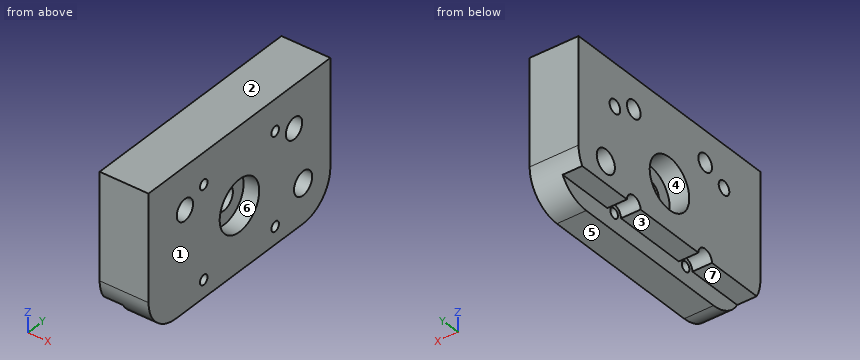
```python
from build123d import *

# Parameters (mm, degrees)
SKETCH_R        = 3.5
SKETCH_R_2      = 6
PAD_DEPTH       = 25
SKETCH001_R     = 5.4
POCKET_DEPTH    = 15
SKETCH002_R     = 13.05
POCKET001_DEPTH = 10
SKETCH006_R     = 2.5
SKETCH006_R_2   = 6
POCKET002_DEPTH = 25
SKETCH005_R     = 4.5
POCKET003_DEPTH = 10
SKETCH007_R     = 13.05
POCKET004_DEPTH = 8
SKETCH009_W     = 120
SKETCH009_H     = 9
POCKET005_DEPTH = 10


with BuildPart() as part:
    # Sketch → Pad (new body)
    with BuildSketch(Plane.YZ):
        with BuildLine():
            Line((-60, -53.999958), (-60, 0))
            Line((-60, 0), (60, 0))
            Line((60, 0), (60, -53.999958))
            ThreePointArc((42.00001, -72), (54.72794, -66.727904), (60, -53.999958))
            Line((-42.00001, -72), (42.00001, -72))
            ThreePointArc((-60, -53.999958), (-54.72794, -66.727904), (-42.00001, -72))
        make_face()
        with Locations((-36, -21.5)):
            Circle(SKETCH_R, mode=Mode.SUBTRACT)
        with Locations((36, -21.5)):
            Circle(SKETCH_R, mode=Mode.SUBTRACT)
        with Locations((0, -39.5)):
            Circle(SKETCH_R_2, mode=Mode.SUBTRACT)
    extrude(amount=PAD_DEPTH)

    # Sketch001 → Pocket (cut)
    with BuildSketch(Plane.YZ.offset(25)):
        with Locations((-36, -21.5)):
            Circle(SKETCH001_R)
        with Locations((36, -21.5)):
            Circle(SKETCH001_R)
    extrude(amount=-POCKET_DEPTH, mode=Mode.SUBTRACT)

    # Sketch002 → Pocket001 (cut)
    with BuildSketch(Plane(origin=(0, 0, 0), x_dir=(0, 1, 0), z_dir=(-1, 0, 0))):
        with Locations((0, 39.5)):
            Circle(SKETCH002_R)
    extrude(amount=-POCKET001_DEPTH, mode=Mode.SUBTRACT)

    # Sketch006 → Pocket002 (cut)
    with BuildSketch(Plane.YZ.offset(25)):
        with Locations((-23.57, -15.93)):
            Circle(SKETCH006_R)
        with Locations((23.57, -15.93)):
            Circle(SKETCH006_R)
        with Locations((-23.57, -63.07)):
            Circle(SKETCH006_R)
        with Locations((23.57, -63.07)):
            Circle(SKETCH006_R)
        with Locations((42, -52)):
            Circle(SKETCH006_R_2)
    extrude(amount=-POCKET002_DEPTH, mode=Mode.SUBTRACT)

    # Sketch005 → Pocket003 (cut)
    with BuildSketch(Plane(origin=(0, 0, 0), x_dir=(0, 1, 0), z_dir=(-1, 0, 0))):
        with Locations((-23.57, 63.07)):
            Circle(SKETCH005_R)
        with Locations((23.57, 63.07)):
            Circle(SKETCH005_R)
        with Locations((-23.57, 15.93)):
            Circle(SKETCH005_R)
        with Locations((23.57, 15.93)):
            Circle(SKETCH005_R)
    extrude(amount=-POCKET003_DEPTH, mode=Mode.SUBTRACT)

    # Sketch007 → Pocket004 (cut)
    with BuildSketch(Plane.YZ.offset(25)):
        with Locations((0, -39.5)):
            Circle(SKETCH007_R)
    extrude(amount=-POCKET004_DEPTH, mode=Mode.SUBTRACT)

    # Sketch009 → Pocket005 (cut)
    with BuildSketch(Plane(origin=(0, 0, 0), x_dir=(0, 1, 0), z_dir=(-1, 0, 0))):
        with Locations((0, 67.5)):
            Rectangle(SKETCH009_W, SKETCH009_H)
    extrude(amount=-POCKET005_DEPTH, mode=Mode.SUBTRACT)


solid = part.part
```
Input: part model. Units: mm. Frame: model coordinates. Face numbers are marked on the shaded views. A direction names the side the tool comes from. Coordinates: 2 decimals unless noted, no trailing zeros. Loops run counter-clockwise (first coordinate to the right, second up) from the corner with the lowest first, then second, coordinate; pieces in that order, holes last. Notation, with made-up numbers: (15.5, -39) - (34.5, -39) arc R14 cw to (34.5, -29) - close; hole circle Ø11 at (2.25, -30.75). An arc over 180 degrees is marked (long way). Answer in a Markdown table with one row per item.
(1) Pin query (flat end, axial travel): P1, Ø5.5, axis at y = 36.5, z = -22, coming from the +X side; P2, Ø8, axis at y = 23.57, z = -15.93, coming from the -X side; P3, Ø1.5, axis at x = 12, z = -55, coming from the -Y side; P4, Ø1.5, axis at x = 4, y = 46.5, coming from the -Z side. Return the tip coordinate at first contact, or that it passes through.
Model answer:
| item | result |
|---|---|
| P1 | passes through |
| P2 | stops at x = 10 |
| P3 | stops at y = -60 |
| P4 | stops at z = -63 |
(2) Cut plane A-A on z = -39.5. Output: boundary loops of the cut face in (x, y), plus the area to 3 significant figures.
Model answer:
| item | result |
|---|---|
| outline | (0, -60) - (25, -60) - (25, -13.05) - (17, -13.05) - (17, -6) - (10, -6) - (10, -13.05) - (0, -13.05) - close; (0, 13.05) - (10, 13.05) - (10, 6) - (17, 6) - (17, 13.05) - (25, 13.05) - (25, 60) - (0, 60) - close |
| area | 2,450 mm² |
(3) Cut plane D-D on x = 6.75. Output: boundary loops of the cut face in (y, z).
Model answer:
| item | result |
|---|---|
| outline | (-60, -54) arc R18 ccw to (-57.59, -63) - (-28.07, -63) arc R4.5 cw to (-19.07, -63) - (19.07, -63) arc R4.5 cw to (28.07, -63) - (57.59, -63) arc R18 ccw to (60, -54) - (60, 0) - (-60, 0) - close; hole circle Ø7 at (-36, -21.5); hole circle Ø9 at (-23.57, -15.93); hole circle Ø26.1 at (0, -39.5); hole circle Ø9 at (23.57, -15.93); hole circle Ø7 at (36, -21.5); hole circle Ø12 at (42, -52) |
(4) Cut plane B-B on y = 0. Output: boundary loops of the cut face in (x, z).
Model answer:
| item | result |
|---|---|
| outline | (0, -63) - (10, -63) - (10, -72) - (25, -72) - (25, -52.55) - (17, -52.55) - (17, -45.5) - (10, -45.5) - (10, -52.55) - (0, -52.55) - close; (0, -26.45) - (10, -26.45) - (10, -33.5) - (17, -33.5) - (17, -26.45) - (25, -26.45) - (25, 0) - (0, 0) - close |
(5) Set-up query: the marked faces 5, 6 and 7. Return all of +Z, -Z, +X, -X, +Y, -Y with unobstructed straight access to the full face (end or side cutting, diameter ignored); none if empty.
Model answer:
| item | result |
|---|---|
| face 5 | -Z, +X, -X, +Y, -Y |
| face 6 | +X |
| face 7 | -Z, -X, +Y, -Y |
(6) Material intervals for L1, parallel to Y at x = 3.5, z = -21.5; L2, parallel to Z at x = 13.75, y = 23.57; L3, parallel to Y at x = 10.5, z = -21, sorted ascending. Write a range as from..to.
Model answer:
| item | result |
|---|---|
| L1 | y = -60..-39.5, -32.5..32.5, 39.5..60 |
| L2 | z = -72..-65.57, -60.57..-18.43, -13.43..0 |
| L3 | y = -60..-41.38, -30.62..30.62, 41.38..60 |
(7) Mould query, pull axis Z, two halves, no side actions, for the marked faces 1, 2, 3 and 4. Classes: pulls with the +Z half, pulls with the -Z half, needs draft (parallel to the pull), parting line crosses it, or undercut.
Model answer:
| item | result |
|---|---|
| face 1 | needs draft |
| face 2 | pulls with the +Z half |
| face 3 | pulls with the -Z half |
| face 4 | undercut |
(8) Cut plane C-C on y = 23.57. Output: boundary loops of the cut face in (x, z).
Model answer:
| item | result |
|---|---|
| outline | (0, -58.57) - (10, -58.57) - (10, -60.57) - (25, -60.57) - (25, -18.43) - (10, -18.43) - (10, -20.43) - (0, -20.43) - close; (0, -11.43) - (10, -11.43) - (10, -13.43) - (25, -13.43) - (25, 0) - (0, 0) - close; (10, -72) - (25, -72) - (25, -65.57) - (10, -65.57) - close |
